Model file for the job. Use its own axes, mm. Round coordinates to 2 decimals unless told otherwise and drop trailing zeros. Loops run counter-clockwise (first coordinate to the right, second up) from the corner with the lowest first, then second, coordinate; pieces in that order, holes last. Notation, with made-up numbers: (85.25, 54.5) - (111.25, 54.5) arc R23 ccw to (111.25, 86.5) - close; hole circle Ø10 at (5.25, 80). An arc over 180 degrees is marked (long way). Use one line per item in the form item = value.
from build123d import *

# Parameters (mm, degrees)
F0_W     = 115.478478
F0_H     = 522.514462
F0_R     = 44.385544
F1_DEPTH = 101.6
F2_SIZE  = 15.24
F3_SIZE  = 15.24
F4_SIZE  = 15.24
F5_SIZE  = 15.24


with BuildPart() as f1:
    # F0 (on Top) → F1 (new body)
    with BuildSketch(Plane.XY):
        Rectangle(F0_W, F0_H)
        with Locations((0, -100.278944)):
            Circle(F0_R, mode=Mode.SUBTRACT)
        with Locations((0.409667, -203.118652)):
            Circle(F0_R, mode=Mode.SUBTRACT)
        Circle(F0_R, mode=Mode.SUBTRACT)
        with Locations((-1.443157, 100.623645)):
            Circle(F0_R, mode=Mode.SUBTRACT)
        with Locations((0, 202.821597)):
            Circle(F0_R, mode=Mode.SUBTRACT)
    extrude(amount=F1_DEPTH)

    # F2
    f2_edges = [f1.edges().sort_by_distance(p)[0] for p in [
        (57.739239, -261.257231, 50.8),
    ]]
    chamfer(f2_edges, length=F2_SIZE)

    # F3
    f3_edges = [f1.edges().sort_by_distance(p)[0] for p in [
        (-57.739239, -261.257231, 50.8),
    ]]
    chamfer(f3_edges, length=F3_SIZE)

    # F4
    f4_edges = [f1.edges().sort_by_distance(p)[0] for p in [
        (57.739239, 261.257231, 50.8),
    ]]
    chamfer(f4_edges, length=F4_SIZE)

    # F5
    f5_edges = [f1.edges().sort_by_distance(p)[0] for p in [
        (-57.739239, 261.257231, 50.8),
    ]]
    chamfer(f5_edges, length=F5_SIZE)


solid = f1.part
1. Cut at C-C, the plane z = 12.5. Give the cut face in (x, y), plus the area to 3 significant figures.
Geometry check:
outline = (-57.74, -246.02) - (-42.5, -261.26) - (42.5, -261.26) - (57.74, -246.02) - (57.74, 246.02) - (42.5, 261.26) - (-42.5, 261.26) - (-57.74, 246.02) - close; hole circle Ø88.77 at (-1.44, 100.62); hole circle Ø88.77 at (0, -100.28); hole circle Ø88.77 at (0, 0); hole circle Ø88.77 at (0, 202.82); hole circle Ø88.77 at (0.41, -203.12)
area = 28,900 mm^2
2. Cut at D-D, the plane y = 191. Give the cut face in (x, z), plus the area to 3 significant figures.
Geometry check:
outline = (-57.74, 0) - (-42.78, 0) - (-42.78, 101.6) - (-57.74, 101.6) - close; (42.78, 0) - (57.74, 0) - (57.74, 101.6) - (42.78, 101.6) - close
area = 3,040 mm^2
3. Pull direction X, two halves, no side cores. Call faces 1 (the flat face through (-50.226, -253.531, 50.089)), 2 (the cylindrical face through (-9.62, 159.49, 50.09)), 3 (the flat face through (51, 4, 0)): +X half, -X half, draft (parallel to the pull), parting line (faces both ways), or undercut.
Geometry check:
face_1 = -X half
face_2 = undercut
face_3 = draft
4. Cut at A-A, the plane y = 0. Give the cut face in (x, z), plus the area to 3 significant figures.
Geometry check:
outline = (-57.74, 0) - (-44.39, 0) - (-44.39, 101.6) - (-57.74, 101.6) - close; (44.39, 0) - (57.74, 0) - (57.74, 101.6) - (44.39, 101.6) - close
area = 2,710 mm^2
5. Cut at B-B, the plane x = -1. Give the cut face in (y, z), plus the area to 3 significant figures.
Geometry check:
outline = (-261.26, 0) - (-247.48, 0) - (-247.48, 101.6) - (-261.26, 101.6) - close; (-158.76, 0) - (-144.65, 0) - (-144.65, 101.6) - (-158.76, 101.6) - close; (-55.9, 0) - (-44.37, 0) - (-44.37, 101.6) - (-55.9, 101.6) - close; (44.37, 0) - (56.24, 0) - (56.24, 101.6) - (44.37, 101.6) - close; (145.01, 0) - (158.45, 0) - (158.45, 101.6) - (145.01, 101.6) - close; (247.2, 0) - (261.26, 0) - (261.26, 101.6) - (247.2, 101.6) - close
area = 8,000 mm^2
6. Wall check: probe 1 along Y at (x, z) = (0, 47) (3 decimals); probe 2 along Y at (x, z) = (6, 42.5); probe 3 along X at (y, z) = (-200, 81.5). Give the ranges that are in metal, low to high.
Geometry check:
probe_1 = -261.257 to -247.502, -158.735 to -144.664, -55.893 to -44.386, 44.386 to 56.262, 144.986 to 158.436, 247.207 to 261.257
probe_2 = -261.26 to -247.15, -159.09 to -144.26, -56.3 to -43.98, 43.98 to 56.87, 144.38 to 158.84, 246.8 to 261.26
probe_3 = -57.74 to -43.87, 44.69 to 57.74
